Autodesk Inventor part; units mm, degrees
ref_plane "YZ Plane" through (0, 0, 0) normal (1, 0, 0) x (0, 1, 0)
ref_plane "XZ Plane" through (0, 0, 0) normal (0, 1, 0) x (-1, 0, 0)
ref_plane "XY Plane" through (0, 0, 0) normal (0, 0, 1) x (1, 0, 0)
sketch "Sketch1" plane through (0, 0, 0) normal (0, 1, 0) x (-1, 0, 0)
  arc A0 (-53.7401, -31.1127) -> (-31.1127, -53.7401) centre (-42.4264, -42.4264) ccw
  arc A1 (31.1127, -53.7401) -> (53.7401, -31.1127) centre (42.4264, -42.4264) ccw
  arc A2 (53.7401, 31.1127) -> (31.1127, 53.7401) centre (42.4264, 42.4264) ccw
  arc A3 (-31.1127, 53.7401) -> (-53.7401, 31.1127) centre (-42.4264, 42.4264) ccw
  line L0 (-53.7401, 31.1127) -> (-33.9411, 11.3137)
  line L1 (11.3137, -33.9411) -> (31.1127, -53.7401)
  line L2 (-53.7401, -31.1127) -> (-33.9411, -11.3137)
  line L3 (11.3137, 33.9411) -> (31.1127, 53.7401)
  line L4 (-31.1127, 53.7401) -> (-11.3137, 33.9411)
  line L5 (33.9411, -11.3137) -> (53.7401, -31.1127)
  line L6 (-31.1127, -53.7401) -> (-11.3137, -33.9411)
  line L7 (33.9411, 11.3137) -> (53.7401, 31.1127)
  arc A4 (11.3137, -33.9411) -> (-11.3137, -33.9411) centre (0, -45.2548) ccw
  arc A5 (33.9411, 11.3137) -> (33.9411, -11.3137) centre (45.2548, 0) ccw
  arc A6 (-11.3137, 33.9411) -> (11.3137, 33.9411) centre (0, 45.2548) ccw
  arc A7 (-33.9411, -11.3137) -> (-33.9411, 11.3137) centre (-45.2548, 0) ccw
  arc A8 (-53.7401, -31.1127) -> (-31.1127, -53.7401) centre (-42.4264, -42.4264) ccw
  arc A9 (31.1127, -53.7401) -> (53.7401, -31.1127) centre (42.4264, -42.4264) ccw
  arc A10 (53.7401, 31.1127) -> (31.1127, 53.7401) centre (42.4264, 42.4264) ccw
  arc A11 (-31.1127, 53.7401) -> (-53.7401, 31.1127) centre (-42.4264, 42.4264) ccw
  line L8 (-53.7401, 31.1127) -> (-33.9411, 11.3137)
  line L9 (11.3137, -33.9411) -> (31.1127, -53.7401)
  line L10 (-53.7401, -31.1127) -> (-33.9411, -11.3137)
  line L11 (11.3137, 33.9411) -> (31.1127, 53.7401)
  line L12 (-31.1127, 53.7401) -> (-11.3137, 33.9411)
  line L13 (33.9411, -11.3137) -> (53.7401, -31.1127)
  line L14 (-31.1127, -53.7401) -> (-11.3137, -33.9411)
  line L15 (33.9411, 11.3137) -> (53.7401, 31.1127)
  arc A12 (11.3137, -33.9411) -> (-11.3137, -33.9411) centre (0, -45.2548) ccw
  arc A13 (33.9411, 11.3137) -> (33.9411, -11.3137) centre (45.2548, 0) ccw
  arc A14 (-11.3137, 33.9411) -> (11.3137, 33.9411) centre (0, 45.2548) ccw
  arc A15 (-33.9411, -11.3137) -> (-33.9411, 11.3137) centre (-45.2548, 0) ccw
  arc A16 (-53.7401, -31.1127) -> (-31.1127, -53.7401) centre (-42.4264, -42.4264) ccw
  arc A17 (31.1127, -53.7401) -> (53.7401, -31.1127) centre (42.4264, -42.4264) ccw
  arc A18 (53.7401, 31.1127) -> (31.1127, 53.7401) centre (42.4264, 42.4264) ccw
  arc A19 (-31.1127, 53.7401) -> (-53.7401, 31.1127) centre (-42.4264, 42.4264) ccw
  line L16 (-53.7401, 31.1127) -> (-33.9411, 11.3137)
  line L17 (11.3137, -33.9411) -> (31.1127, -53.7401)
  line L18 (-53.7401, -31.1127) -> (-33.9411, -11.3137)
  line L19 (11.3137, 33.9411) -> (31.1127, 53.7401)
  line L20 (-31.1127, 53.7401) -> (-11.3137, 33.9411)
  line L21 (33.9411, -11.3137) -> (53.7401, -31.1127)
  line L22 (-31.1127, -53.7401) -> (-11.3137, -33.9411)
  line L23 (33.9411, 11.3137) -> (53.7401, 31.1127)
  arc A20 (11.3137, -33.9411) -> (-11.3137, -33.9411) centre (0, -45.2548) ccw
  arc A21 (33.9411, 11.3137) -> (33.9411, -11.3137) centre (45.2548, 0) ccw
  arc A22 (-11.3137, 33.9411) -> (11.3137, 33.9411) centre (0, 45.2548) ccw
  arc A23 (-33.9411, -11.3137) -> (-33.9411, 11.3137) centre (-45.2548, 0) ccw
  point P0 (0, 0)
  point P1 (0, 0)
  point P2 (0, 0)
  point P3 (0, 0)
  point P4 (0, 0)
  point P5 (0, 0)
  point P6 (0, 0)
extrude "Extrusion1" add sketch "Sketch1" along normal blind 2
sketch "Sketch2" plane through (0, 0, 0) normal (0, -1, 0) x (1, 0, 0)
  circle A0 centre (0, 0) radius 3
  dimension "d2" = 6
extrude "Extrusion2" cut sketch "Sketch2" against normal blind 30
sketch "Sketch3" plane through (0, 2, 0) normal (0, 1, 0) x (1, 0, 0)
  arc A0 (53.7401, 31.1127) -> (31.1127, 53.7401) centre (42.4264, 42.4264) ccw
  circle A1 centre (42.4264, 42.4264) radius 1.5
  arc A2 (-31.1127, 53.7401) -> (-53.7401, 31.1127) centre (-42.4264, 42.4264) ccw
  circle A3 centre (-42.4264, 42.4264) radius 1.5
  arc A4 (-53.7401, -31.1127) -> (-31.1127, -53.7401) centre (-42.4264, -42.4264) ccw
  circle A5 centre (-42.4264, -42.4264) radius 1.5
  arc A6 (31.1127, -53.7401) -> (53.7401, -31.1127) centre (42.4264, -42.4264) ccw
  circle A7 centre (42.4264, -42.4264) radius 1.5
  line L0 (0, 0) -> (28, 0) construction
  circle A8 centre (-19.799, 19.799) radius 1.5
  circle A9 centre (19.799, 19.799) radius 1.5
  circle A10 centre (19.799, -19.799) radius 1.5
  circle A11 centre (-19.799, -19.799) radius 1.5
  dimension "d5" = 3
  dimension "d6" = 3
  dimension "d7" = 3
  dimension "d8" = 3
  dimension "d11" = 3
  dimension "d12" = 3
  dimension "d13" = 3
  dimension "d14" = 3
extrude "Extrusion3" cut sketch "Sketch3" against normal blind 20
sketch "Sketch4" plane through (0, 2, 0) normal (0, 1, 0) x (1, 0, 0)
  line L0 (-7.4916, -30.1191) -> (-44.7907, -22.1777)
  line L1 (-8.9058, -31.5333) -> (-7.4916, -30.1191)
  line L2 (-44.7907, -22.1777) -> (-46.2121, -23.5847)
  line L3 (-7.4916, -30.1191) -> (-8.9058, -31.5333)
  line L4 (-8.9058, -31.5333) -> (-46.2121, -23.5847)
  line L5 (7.4916, 30.1191) -> (44.7907, 22.1777)
  line L6 (8.9058, 31.5333) -> (7.4916, 30.1191)
  line L7 (44.7907, 22.1777) -> (46.2121, 23.5847)
  line L8 (7.4916, 30.1191) -> (8.9058, 31.5333)
  line L9 (8.9058, 31.5333) -> (46.2121, 23.5847)
  line L10 (45.2798, -22.6524) -> (41.4801, -40.5283)
  line L11 (41.4801, -40.5283) -> (43.4364, -40.9441)
  line L12 (46.966, -24.3386) -> (43.4364, -40.9441)
  line L13 (46.966, -24.3386) -> (45.2798, -22.6524)
  line L14 (-45.2798, 22.6524) -> (-41.4801, 40.5283)
  line L15 (-46.966, 24.3386) -> (-45.2798, 22.6524)
  line L16 (-46.966, 24.3386) -> (-43.4364, 40.9441)
  line L17 (-41.4801, 40.5283) -> (-43.4364, 40.9441)
  point P0 (0, 0)
  dimension "d20" = 2
  dimension "d21" = 2
  dimension "d24" = 360
  dimension "d27" = 2
  dimension "d31" = 360
extrude "Extrusion4" [suppressed]
sketch "Sketch7" plane through (0, 2, 0) normal (0, 1, 0) x (1, 0, 0)
  line L0 (0, 0) -> (44, 0) construction
  circle A0 centre (31.1127, -31.1127) radius 1.5
  circle A1 centre (31.1127, 31.1127) radius 1.5
  circle A2 centre (-31.1127, 31.1127) radius 1.5
  circle A3 centre (-31.1127, -31.1127) radius 1.5
  dimension "d48" = 3
  dimension "d51" = 360
extrude "Extrusion7" cut sketch "Sketch7" against normal blind 10
properties part number "platform 1"
CAD build for the part. Positions are in the model's coordinates, mm. A direction names the side the tool comes from. Round coordinates to 2 decimals unless told otherwise and drop trailing zeros. Loops run counter-clockwise (first coordinate to the right, second up) from the corner with the lowest first, then second, coordinate; pieces in that order, holes last. Notation, with made-up numbers: (-15.75, 70.25) - (13.25, 70.25) arc R21 cw to (13.25, 76.25) - close; hole circle Ø8 at (40, 11.25). An arc over 180 degrees is marked (long way). Put each result on its own line as item: value.
1. Two-plate mould, pull along Z, no slides. Class faces 4 (the flat face through (21.35, 0.99, -43.98)), 5 (the flat face through (21.35, 0.99, 43.98)), 6 (the cylindrical face through (-53.986, 0.986, -53.489)), 7 (the cylindrical face through (-21.298, 1.014, 19.733)): released by +Z, released by -Z, zero draft, split by the parting line, or undercut.
Geometry check:
face 4: released by -Z
face 5: released by +Z
face 6: undercut
face 7: undercut
2. Slice it at A-A on x = 0. List the corners of the cut face in (y, z), and give its area (3 significant figures).
Geometry check:
outline: (0, -29.25) - (2, -29.25) - (2, -3) - (0, -3) - close; (0, 3) - (2, 3) - (2, 29.25) - (0, 29.25) - close
area: 105 mm²
3. 3-axis set-ups, long thin cutter, end or side, ignore diameter. For faces 1 (the flat face through (43.98, 0.99, -21.35)), 2 (the flat face through (1, 2, 14)), 3 (the flat face through (-43.7, 0.99, -21.07)): which of +Z, -Z, +X, -X, +Y, -Y reach the whole face in a straight line?
Geometry check:
face 1: +X, +Y, -Y
face 2: +Z, -Z, +X, -X, +Y
face 3: -X, +Y, -Y
4. Slice it at D-D on z = -26. List the corners of the cut face in (x, y).
Geometry check:
outline: (-48.63, 0) - (48.63, 0) - (48.63, 2) - (-48.63, 2) - close
5. Pin check, flat tips, straight feed: P1, Ø2.5, axis at x = 31.11, z = -31.11, coming from the +Y side; P2, Ø1, axis at y = 1.5, z = 19, coming from the +X side; P3, Ø1, axis at x = 10.5, y = 1.5, coming from the +Z side. Stop position of each tip, or through.
Geometry check:
P1: through
P2: x = 42.13
P3: z = 33.64
6. Slice it at B-B on z = 0. List the corners of the cut face in (x, y).
Geometry check:
outline: (-29.25, 0) - (-3, 0) - (-3, 2) - (-29.25, 2) - close; (3, 0) - (29.25, 0) - (29.25, 2) - (3, 2) - close
7. Wall check: line 1 (Z direction, x = 0, y = 1.15); line 2 (Z direction, x = -31, y = 1.05); line 3 (X direction, y = 1.4, z = -19). Give the ranges that are in metal, low to high.
Geometry check:
line 1: -29.25 to -3, 3 to 29.25
line 2: -53.63 to -32.61, -29.62 to -7.27, 7.27 to 29.62, 32.61 to 53.63
line 3: -41.63 to -21.07, -18.53 to 18.53, 21.07 to 41.63
8. Slice it at C-C on y = 1.55. Give the number of separate pieces and of enclosed holes in the cut face, and give its area (3 significant figures).
Geometry check:
separate pieces: 1
enclosed holes: 13
area: 8,370 mm²
